Can you work these out from the drawing? Everything is in mm from the part's minimum corner. A direction names the side the tool comes from. Coordinates: 2 decimals unless noted, no trailing zeros. Order: outer loops, then holes, each group sorted by start corner. A loop starts at its lowest first (then second) coordinate and runs counter-clockwise, first axis right, second up. Notation, with made-up numbers: M 23.5,74 L 44.5,74 A31 ccw 44.5,98 Z; hole C 57,82 d7. An arc over 180 degrees is marked long. Answer as a JSON object with one key per item and string values.
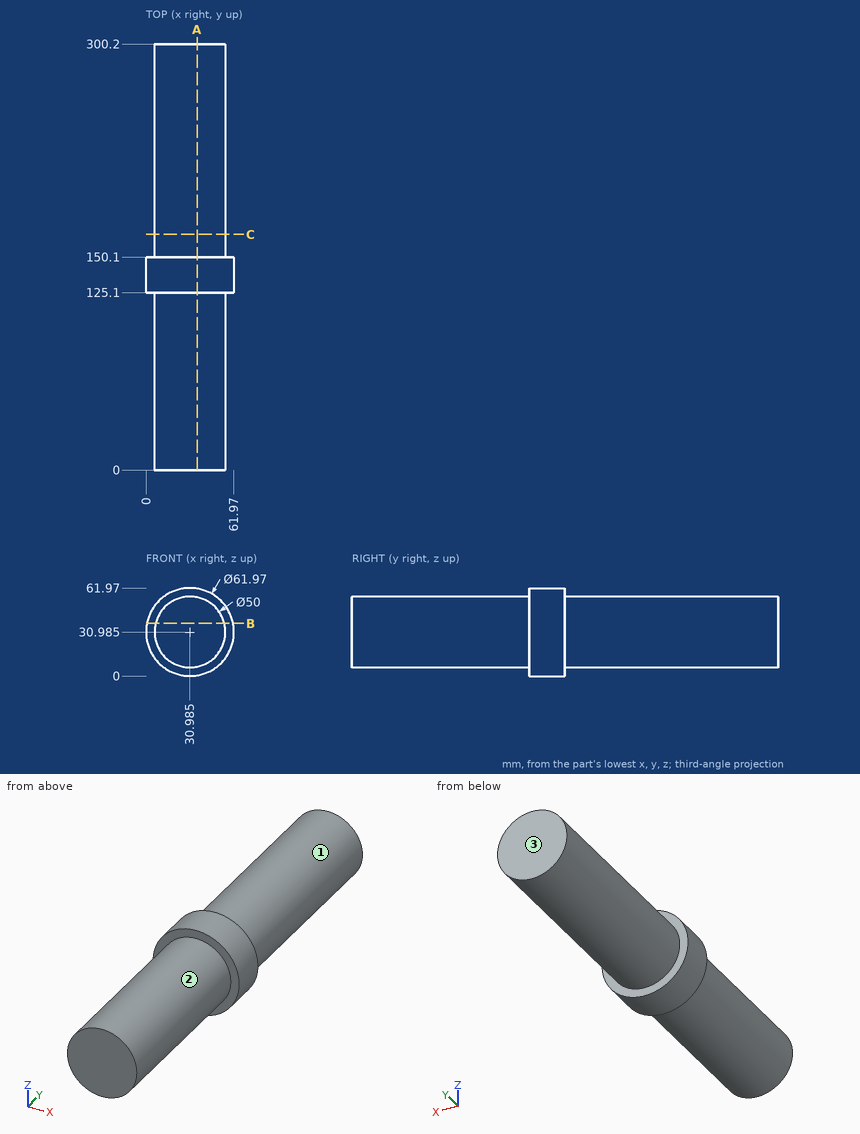
Item 1: I want a section at A-A, the plane x = 36. Write out the boundary of the cut face in (y, z), plus the area to 3 significant figures.
Answers follow:
{"outline": "M 0,6.49 L 125.1,6.49 L 125.1,0.41 L 150.1,0.41 L 150.1,6.49 L 300.2,6.49 L 300.2,55.48 L 150.1,55.48 L 150.1,61.56 L 125.1,61.56 L 125.1,55.48 L 0,55.48 Z", "area": "15,000 mm^2"}
Item 2: Please list where these lines run through material, in increasing order: line 1 (Y direction, x = 54, z = 45.5); line 2 (X direction, y = 89.5, z = 53); line 3 (Z direction, x = 10, y = 34.5).
Answers follow:
{"line 1": "y = 125.1 to 150.1", "line 2": "x = 19.14 to 42.83", "line 3": "z = 17.4 to 44.57"}
Item 3: I want a section at B-B, the plane z = 37. Write out the boundary of the cut face in (x, y).
Answers follow:
{"outline": "M 0.59,125.1 L 6.72,125.1 L 6.72,0 L 55.25,0 L 55.25,125.1 L 61.38,125.1 L 61.38,150.1 L 55.25,150.1 L 55.25,300.2 L 6.72,300.2 L 6.72,150.1 L 0.59,150.1 Z"}
Item 4: I want a section at C-C, the plane y = 166. Write out the boundary of the cut face in (x, z) (3 decimals), plus the area to 3 significant figures.
Answers follow:
{"outline": "C 30.985,30.985 d50", "area": "1,960 mm^2"}
Item 5: Which directions (+Z, -Z, +X, -X, +Y, -Y) give clear straight access to the entire face, cutting with the end or side of a thin tool? Please do the marked faces 1, 2 and 3.
Answers follow:
{"face 1": "+Y", "face 2": "-Y", "face 3": "+Z, -Z, +X, -X, +Y"}
Item 6: I'm going to push flat-ended pins straight in: pin 1 (10 mm diameter, centred on x = 35.5, y = 196, fed in from +Z) (3 decimals); pin 2 (3 mm diameter, centred on x = 51.5, y = 215, fed in from -Z); pin 3 (8 mm diameter, centred on y = 89, z = 22, fed in from +X). Where does each tip first touch, or does it pass through?
Answers follow:
{"pin 1": "stops at z = 55.985", "pin 2": "stops at z = 14.75", "pin 3": "stops at x = 55.48"}
